Study the drawing (mm; zero at the part's minimum x, y, z) and answer. A direction names the side the tool comes from. Give positions to 0.01 mm unless a question says otherwise; leave off trailing zeros. Write each loop counter-clockwise with the first axis right and the second up, starting at its lowest first coordinate (ties: lowest second). Pieces come first, ordered by that corner, then holes. Notation, with made-up numbers: M 20.5,-17.75 L 46.5,-17.75 A24 ccw 46.5,-6.75 Z; hole C -38.75,43 d9. An arc over 180 degrees is marked long. Use a Markdown table: item, result. Add a question column.
Item 1: Consider probe 1 along X at (y, z) = (74.22, 17.5); probe 2 along Y at (x, z) = (17.46, 9.8). Determine where each line is inside the solid, lowest interval first. Write a range as [from, to].
Item 2: The mould has two halves that part along Y. Classify the marked faces 3, 4 and 5: pulls with the +Y half, pulls with the -Y half, needs draft (parallel to the pull), parting line crosses it, or undercut.
Item 3: A cutting plane is placed at A-A on z = 19.75. Determine the outline of the cut face in (x, y), then the cut area to 3 significant figures.
Item 4: Given P1, Ø5.5, axis at x = 19, y = 12, coming from the +Z side; P2, Ø1.8, axis at x = 60.76, y = 12.36, coming from the +Z side; P3, Ø1, axis at y = 58.5, z = 12.5, coming from the -X side, each flat-ended and moving along its own axis, determine where each tip first touches the part or whether it passes through.
Item 5: A cutting plane is placed at B-B on x = 74.22. Determine the outline of the cut face in (y, z), then the cut area to 3 significant figures.
Item 6: A cutting plane is placed at C-C on y = 44. Determine the outline of the cut face in (x, z), then the cut area to 3 significant figures.
Item 7: For the marked faces 1 and 2, determine the directions among +Z, -Z, +X, -X, +Y, -Y from which every point of the face is accessible in a straight line to the end or side of a thin tool.
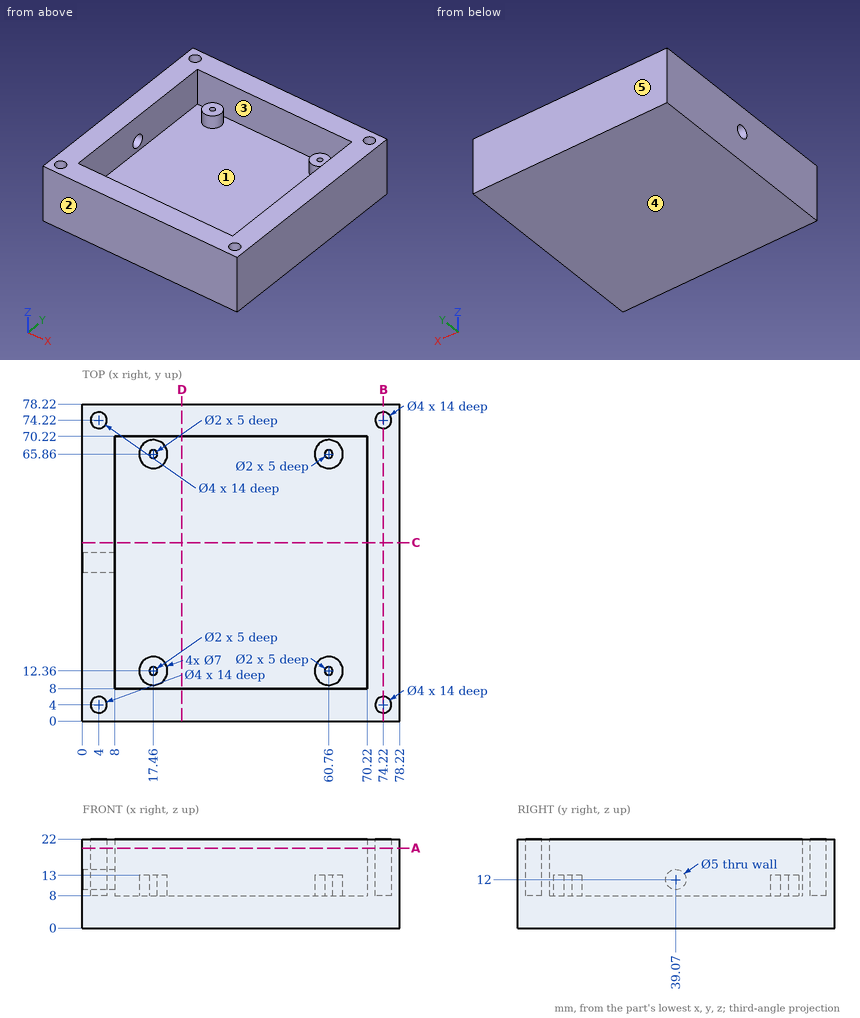
Filled in:
| question | item | result |
|---|---|---|
| 1 | probe 1 | [0, 2], [6, 72.22], [76.22, 78.22] |
| 1 | probe 2 | [0, 8], [8.86, 11.36], [13.36, 15.86], [62.36, 64.86], [66.86, 69.36], [70.22, 78.22] |
| 2 | face 3 | undercut |
| 2 | face 4 | needs draft |
| 2 | face 5 | pulls with the +Y half |
| 3 | outline | M 0,0 L 78.22,0 L 78.22,78.22 L 0,78.22 Z; hole C 4,4 d4; hole C 4,74.22 d4; hole M 8,8 L 70.22,8 L 70.22,70.22 L 8,70.22 Z; hole C 74.22,4 d4; hole C 74.22,74.22 d4 |
| 3 | area | 2,200 mm² |
| 4 | P1 | z = 13 |
| 4 | P2 | z = 8 |
| 4 | P3 | x = 0 |
| 5 | outline | M 0,0 L 78.22,0 L 78.22,22 L 76.22,22 L 76.22,8 L 72.22,8 L 72.22,22 L 6,22 L 6,8 L 2,8 L 2,22 L 0,22 Z |
| 5 | area | 1,610 mm² |
| 6 | outline | M 0,0 L 78.22,0 L 78.22,22 L 70.22,22 L 70.22,8 L 8,8 L 8,22 L 0,22 Z |
| 6 | area | 850 mm² |
| 7 | face 1 | +Z |
| 7 | face 2 | +Z, -Z, +X, -X, -Y |
